The model under review builds one solid part; all positions refer to its coordinate system, in mm. A direction names the side the tool comes from. Round coordinates to 2 decimals unless told otherwise and drop trailing zeros. Write each loop counter-clockwise with the first axis right and the second up, starting at its lowest first coordinate (ties: lowest second). Pieces come first, ordered by that corner, then holes. Notation, with made-up numbers: (73, 59.25) - (93, 59.25) arc R14 cw to (93, 69.25) - close; hole circle Ø1 at (71, 19). An arc over 180 degrees is marked (long way). Return JSON: item names as keys, results as strings.
from build123d import *

# Parameters (mm, degrees)
SKETCH015_R  = 1.55
PAD012_DEPTH = 0.75
FILLET016_R  = 0.4
FILLET017_R  = 1


with BuildPart() as part:
    # Sketch015 → Pad012 (new body, symmetric)
    with BuildSketch(Plane.XZ):
        with BuildLine():
            Line((-20, 10), (-20, -7))
            Line((-20, -8.5), (-20, -7))
            Line((-20, -8.5), (-20, -10))
            Line((-20, -10), (20, -10))
            Line((20, -10), (20, 6.5))
            Line((18.133975, 7), (20, 6.5))
            Line((18.133975, 7), (-14.2, 7))
            ThreePointArc((-15, 7), (-14.6, 6.6), (-14.2, 7))
            Line((-15, 7), (-15, 7.7))
            ThreePointArc((-15, 8.5), (-15.4, 8.1), (-15, 7.7))
            Line((-15, 8.5), (18.133975, 8.5))
            Line((18.133975, 8.5), (20, 9))
            Line((20, 9), (20, 10))
            Line((20, 10), (-20, 10))
        make_face()
        Circle(SKETCH015_R, mode=Mode.SUBTRACT)
    extrude(amount=PAD012_DEPTH, both=True)

    # Fillet016
    fillet016_edges = [part.edges().sort_by_distance(p)[0] for p in [
        (-15, 0, 7.7),
        (-14.2, 0, 7),
        (20, 0, 9),
        (20, 0, 10),
    ]]
    fillet(fillet016_edges, radius=FILLET016_R)

    # Fillet017
    fillet017_edges = [part.edges().sort_by_distance(p)[0] for p in [
        (-20, 0, 10),
        (-20, 0, -10),
        (20, 0, -10),
        (20, 0, 6.5),
        (18.133975, 0, 7),
        (18.133975, 0, 8.5),
    ]]
    fillet(fillet017_edges, radius=FILLET017_R)


solid = part.part
(1) Add section B-B (x = 0). Write out the cut boundary in (y, z), plus the area to 3 significant figures.
Filled in:
{"outline": "(-0.75, -10) - (0.75, -10) - (0.75, -1.55) - (-0.75, -1.55) - close; (-0.75, 1.55) - (0.75, 1.55) - (0.75, 7) - (-0.75, 7) - close; (-0.75, 8.5) - (0.75, 8.5) - (0.75, 10) - (-0.75, 10) - close", "area": "23.1 mm2"}
(2) Add section D-D (x = 4). Write out the cut boundary in (y, z), plus the area to 4 significant figures.
Filled in:
{"outline": "(-0.75, -10) - (0.75, -10) - (0.75, 7) - (-0.75, 7) - close; (-0.75, 8.5) - (0.75, 8.5) - (0.75, 10) - (-0.75, 10) - close", "area": "27.75 mm2"}
(3) Add section A-A (y = 0.1). Write out the cut boundary in (x, z), plus the area to 3 significant figures.
Filled in:
{"outline": "(-20, -9) arc R1 ccw to (-19, -10) - (19, -10) arc R1 ccw to (20, -9) - (20, 5.73) arc R1 ccw to (19.26, 6.7) - (18.26, 6.97) arc R1 ccw to (18, 7) - (-13.91, 7) arc R0.4 ccw to (-14.25, 6.8) arc R0.4 cw to (-15, 7) - (-15, 7.41) arc R0.4 ccw to (-15.2, 7.75) arc R0.4 cw to (-15, 8.5) - (18, 8.5) arc R1 ccw to (18.26, 8.53) - (19.7, 8.92) arc R0.4 ccw to (20, 9.31) - (20, 9.6) arc R0.4 ccw to (19.6, 10) - (-19, 10) arc R1 ccw to (-20, 9) - close; hole circle Ø3.1 at (0, 0)", "area": "738 mm2"}
(4) Wall thickness on line 1 (Z direction, x = 0, y = 0.1); line 2 (Z direction, x = 12.5, y = 0.6); line 3 (X direction, y = -0.55, z = 0.5): over which ranges is each line inside the solid? List them lowest first.
Filled in:
{"line 1": "z = -10 to -1.55, 1.55 to 7, 8.5 to 10", "line 2": "z = -10 to 7, 8.5 to 10", "line 3": "x = -20 to -1.47, 1.47 to 20"}
(5) Mouldability with a two-part tool opening along Z and no side actions: class faces 1 (the flat face through (1, 0, 8.5)), 2 (the flat face through (0, 0, -10)), 3 (the cylindrical face through (-19.699, 0.01, 9.715)) as released by +Z, released by -Z, zero draft, split by the parting line, or undercut.
Filled in:
{"face 1": "undercut", "face 2": "released by -Z", "face 3": "released by +Z"}
(6) Add section C-C (z = 0). Write out the cut boundary in (x, y).
Filled in:
{"outline": "(-20, -0.75) - (-1.55, -0.75) - (-1.55, 0.75) - (-20, 0.75) - close; (1.55, -0.75) - (20, -0.75) - (20, 0.75) - (1.55, 0.75) - close"}
(7) For faces 4 (the flat face through (1, 0, 10)), 5 (the flat face through (18.972, -0.01, 8.725)), list the 3-axis set-ups (+Z, -Z, +X, -X, +Y, -Y) from which the entire face can be reached by the end or side of a thin tool; tool diameter is ignored.
Filled in:
{"face 4": "+Z, +X, -X, +Y, -Y", "face 5": "+X, +Y, -Y"}
(8) Clearance check with a flat-ended pin moving along its axis: pin 1 Ø5 at (x, z) = (0, 0) entering from -Y. State where the tip first meets the part, or that it passes through.
Filled in:
{"pin 1": "stops at y = -0.75"}
